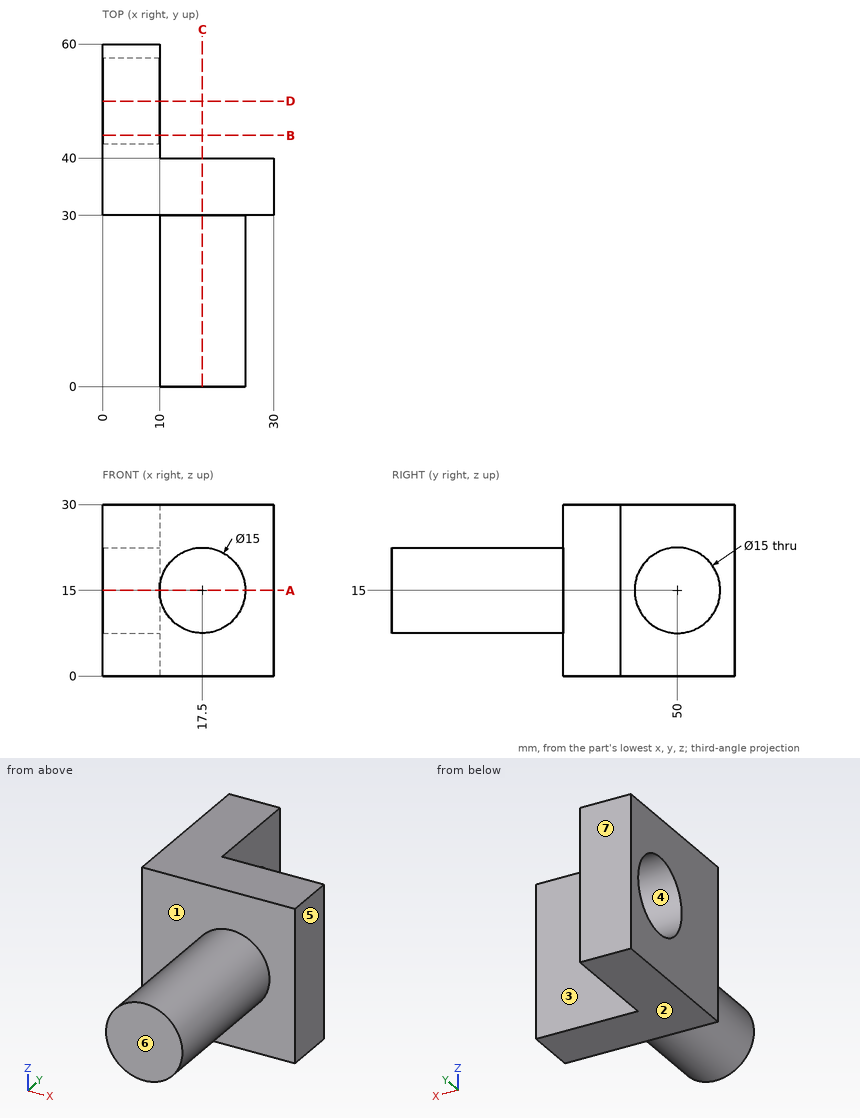
Source: three-view drawing plus pictorial views. Frame: mm from the lowest corner of the part. A direction names the side the tool comes from. Coordinates: 2 decimals unless noted, no trailing zeros. Order: outer loops, then holes, each group sorted by start corner. A loop starts at its lowest first (then second) coordinate and runs counter-clockwise, first axis right, second up. Notation, with made-up numbers: M 2.5,78 L 59.5,78 A12 cw 59.5,99 Z; hole C 14.5,-0.5 d9. An arc over 180 degrees is marked long. One line per question, with ' | ' between items.
Item 1: Section C-C (x = 17.5). Output: boundary loops of the cut face in (y, z), then the cut area to 3 significant figures.
Geometry results:
outline: M 0,7.5 L 30,7.5 L 30,0 L 40,0 L 40,30 L 30,30 L 30,22.5 L 0,22.5 Z | area: 750 mm^2
Item 2: Pin query (flat end, axial travel): pin 1 (1 mm diameter, centred on x = 24, y = 9, fed in from -Z); pin 2 (17 mm diameter, centred on y = 50, z = 15, fed in from +X); pin 3 (4 mm diameter, centred on x = 20, z = 20.5, fed in from +Y). Return the tip coordinate at first contact, or that it passes through.
Geometry results:
pin 1: stops at z = 10.5 | pin 2: stops at x = 10 | pin 3: stops at y = 40
Item 3: Draft query along Y for the marked faces 4, 5, 6 and 7. Return one class per face: released by +Y, released by -Y, zero draft, split by the parting line, or undercut.
Geometry results:
face 4: undercut | face 5: zero draft | face 6: released by -Y | face 7: released by +Y
Item 4: Section B-B (y = 44). Output: boundary loops of the cut face in (x, z), then the cut area to 3 significant figures.
Geometry results:
outline: M 0,0 L 10,0 L 10,10.5 L 0,10.5 Z; M 0,19.5 L 10,19.5 L 10,30 L 0,30 Z | area: 210 mm^2
Item 5: Section A-A (z = 15). Output: boundary loops of the cut face in (x, y).
Geometry results:
outline: M 0,30 L 10,30 L 10,0 L 25,0 L 25,30 L 30,30 L 30,40 L 10,40 L 10,42.5 L 0,42.5 Z; M 0,57.5 L 10,57.5 L 10,60 L 0,60 Z
Item 6: Ray query, line 1 along Z through (x, y) = (6.25, 50); line 2 along X through (y, z) = (44, 4.25); line 3 along Y through (x, z) = (2.75, 12.75). Return the intervals inside material, ascending.
Geometry results:
line 1: z = 0 to 7.5, 22.5 to 30 | line 2: x = 0 to 10 | line 3: y = 30 to 42.85, 57.15 to 60
Item 7: Reachability of the marked faces 1, 2 and 3 from +Z, -Z, +X, -X, +Y, -Y: full face, straight path, thin tool, end or side. Return the list, or none.
Geometry results:
face 1: -Y | face 2: -Z, +X, -X, +Y, -Y | face 3: +Z, -Z, +X, +Y
Item 8: Section D-D (y = 50). Output: boundary loops of the cut face in (x, z).
Geometry results:
outline: M 0,0 L 10,0 L 10,7.5 L 0,7.5 Z; M 0,22.5 L 10,22.5 L 10,30 L 0,30 Z
